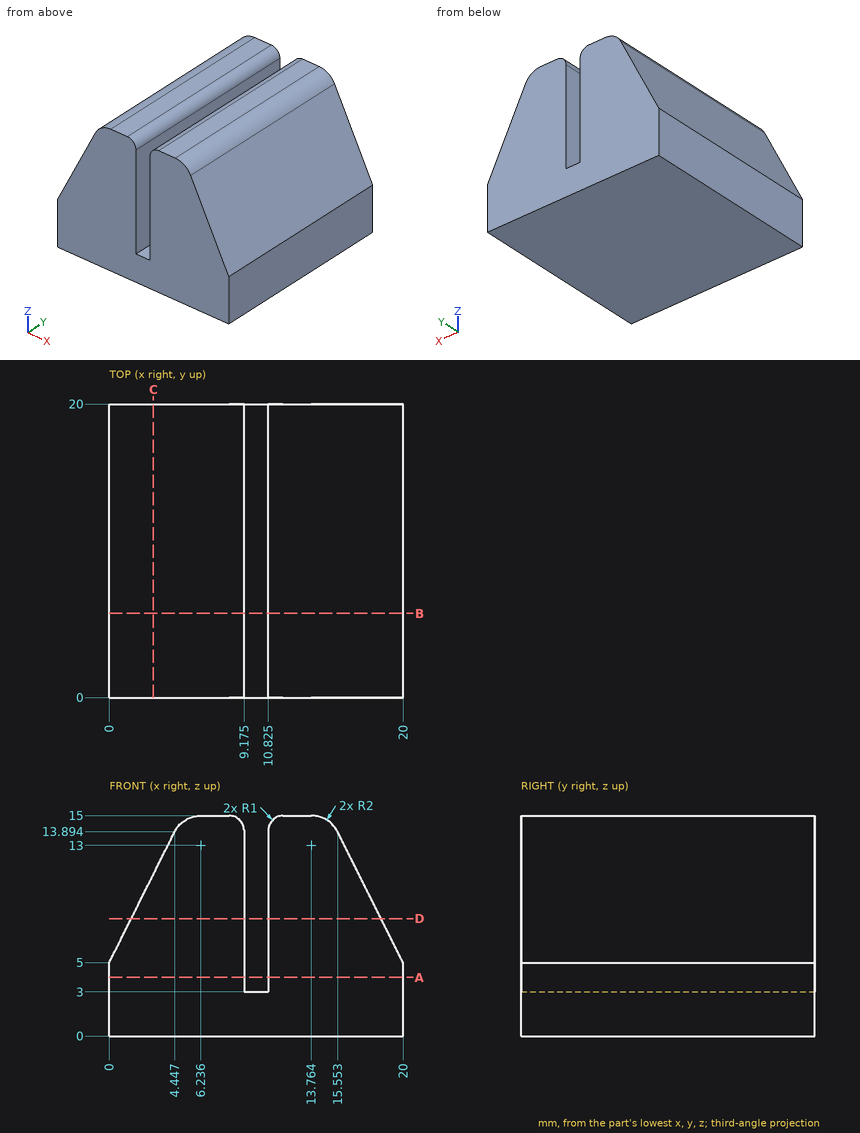
The drawing under review shows one solid part. Ordinate dimensions are in mm from its lowest x, y, z. Round coordinates to 2 decimals unless told otherwise and drop trailing zeros. Order: outer loops, then holes, each group sorted by start corner. A loop starts at its lowest first (then second) coordinate and runs counter-clockwise, first axis right, second up. Notation, with made-up numbers: (-13, -37) -> (38, -37) arc R15 cw to (38, -22) -> close; hole circle Ø5 at (73.5, 67.25). An arc over 180 degrees is marked (long way). Use a Markdown table: item, result.
Q1. We need section C-C on x = 3. Write out the cut boundary in (y, z), then the cut area to 3 significant figures.
Values:
| item | result |
|---|---|
| outline | (0, 0) -> (20, 0) -> (20, 11) -> (0, 11) -> close |
| area | 220 mm^2 |
Q2. Clearance check with flat-ended pins moving along their axes: P1, Ø3.5, axis at y = 9, z = 7, coming from the +X side (1 decimal); P2, Ø4, axis at y = 11, z = 7.5, coming from the -X side; P3, Ø0.8, axis at x = 10, y = 14, coming from the +Z side; P4, Ø4, axis at x = 16, y = 16.5, coming from the -Z side. State where each tip first meets the part, or that it passes through.
Values:
| item | result |
|---|---|
| P1 | stops at x = 19.9 |
| P2 | stops at x = 0.25 |
| P3 | stops at z = 3 |
| P4 | stops at z = 0 |
Q3. We need section A-A on z = 4. Write out the cut boundary in (x, y) (1 decimal).
Values:
| item | result |
|---|---|
| outline | (0, 0) -> (9.2, 0) -> (9.2, 20) -> (0, 20) -> close; (10.8, 0) -> (20, 0) -> (20, 20) -> (10.8, 20) -> close |
Q4. We need section D-D on z = 8. Write out the cut boundary in (x, y) (1 decimal), then the cut area to 3 significant figures.
Values:
| item | result |
|---|---|
| outline | (1.5, 0) -> (9.2, 0) -> (9.2, 20) -> (1.5, 20) -> close; (10.8, 0) -> (18.5, 0) -> (18.5, 20) -> (10.8, 20) -> close |
| area | 307 mm^2 |
Q5. For line 1 (X direction, y = 15, z = 11.75) (1 decimal); line 2 (X direction, y = 5.25, z = 13.25) (1 decimal); line 3 (Z direction, x = 9.75, y = 17), list the stretches that pass through material, from the lowest coordinate up.
Values:
| item | result |
|---|---|
| line 1 | x = 3.4 to 9.2, 10.8 to 16.6 |
| line 2 | x = 4.1 to 9.2, 10.8 to 15.9 |
| line 3 | z = 0 to 3 |
Q6. We need section B-B on y = 5.75. Write out the cut boundary in (x, z) (1 decimal).
Values:
| item | result |
|---|---|
| outline | (0, 0) -> (20, 0) -> (20, 5) -> (15.6, 13.9) arc R2 ccw to (13.8, 15) -> (11.8, 15) arc R1 ccw to (10.8, 14) -> (10.8, 3) -> (9.2, 3) -> (9.2, 14) arc R1 ccw to (8.2, 15) -> (6.2, 15) arc R2 ccw to (4.4, 13.9) -> (0, 5) -> close |
